Can you work these out from the model? Positions are in its coordinate system, mm. A direction names the side the tool comes from. Round coordinates to 2 decimals unless told otherwise and drop trailing zeros. Order: outer loops, then holes, each group sorted by start corner. A loop starts at its lowest first (then second) coordinate and runs counter-clockwise, first axis right, second up.
Q1. For faces 1 (the face through (16.051, 0.507, -3.636)), 2 (the face through (-3.905, 1.812, -0.867)), 3 (the face through (10, 0, 1)), which set-ups out of +Z, -Z, +X, -X, +Y, -Y let a thin tool reach every point of the face, with its end or its side?
Q2. Will these pins go through, and if not, where does the flat tip stop? P1, Ø1, axis at y = 2, z = 2.5, coming from the -X side; P2, Ø1.5, axis at y = 2.5, z = -3, coming from the -X side; P3, Ø4, axis at x = 9.5, z = 3, coming from the -Y side; P4, Ø1.5, axis at y = 0.5, z = -2, coming from the -X side.
Q3. If we section it at A-A (y = 1.4): Please give me the cut outline in (x, z).
Q4. If we section it at C-C (x = 5.25): Please give me the cut outline in (y, z), plus the area to 3 significant figures.
Q5. If I drill on line 1 (Y direction, x = 7.75, z = 1.5); line 2 (X direction, y = 1.7, z = -0.5); line 3 (Z direction, x = 9.75, y = 0.65), over which ranges is the centre line in solid material (lowest first)?
Q6. We'd pull the mould along X, two halves only. Please class faces 4 (the face through (1.3, 0.5, -4)), 5 (the face through (9.9, 0.5, 0)): pulls with the +X half, pulls with the -X half, needs draft (parallel to the pull), parting line crosses it, or undercut.
Q7. If we section it at B-B (x = 11.75): Please give me the cut outline in (y, z), plus the area to 3 significant figures.
from build123d import *

# Parameters (mm, degrees)
SKETCH1_R             = 4
BOSS_EXTRUDE1_DEPTH   = 4
BOSS_EXTRUDE1_2_DEPTH = 4
FILLET1_R             = 1
FILLET2_R             = 1
SKETCH2_W             = 20
SKETCH2_H             = 8
BOSS_EXTRUDE2_DEPTH   = 1
SKETCH3_R             = 6
CUT_EXTRUDE1_DEPTH    = 1
FILLET3_R             = 3


with BuildPart() as part:
    # Sketch1 → Boss-Extrude1 (new body)
    with BuildSketch(Plane(origin=(0, 0, 0), x_dir=(1, 0, 0), z_dir=(0, 1, 0))):
        with Locations(Location((0, 0, 0), (0, 0, 270))):
            Circle(SKETCH1_R)
    extrude(amount=BOSS_EXTRUDE1_DEPTH)

    # Fillet1
    fillet1_edges = [part.edges().sort_by_distance(p)[0] for p in [
        (0, 4, -4),
    ]]
    fillet(fillet1_edges, radius=FILLET1_R)



with BuildPart() as body_2:
    # Sketch1 → Boss-Extrude1 2 (new body)
    with BuildSketch(Plane(origin=(0, 0, 0), x_dir=(1, 0, 0), z_dir=(0, 1, 0))):
        with Locations(Location((20, 0, 0), (0, 0, 270))):
            Circle(SKETCH1_R)
    extrude(amount=BOSS_EXTRUDE1_2_DEPTH)

    # Fillet2
    fillet2_edges = [body_2.edges().sort_by_distance(p)[0] for p in [
        (20, 4, -4),
    ]]
    fillet(fillet2_edges, radius=FILLET2_R)


with BuildPart() as part_1:
    add(part.part)

    add(body_2.part)  # Boss-Extrude2 merges body 2
    # Sketch2 → Boss-Extrude2 (add)
    with BuildSketch(Plane(origin=(0, 0, 0), x_dir=(-1, 0, 0), z_dir=(0, -1, 0))):
        with Locations((-10, 0)):
            Rectangle(SKETCH2_W, SKETCH2_H)
    extrude(amount=-BOSS_EXTRUDE2_DEPTH)

    # Sketch3 → Cut-Extrude1 (cut)
    with BuildSketch(Plane(origin=(0, 1, 0), x_dir=(1, 0, 0), z_dir=(0, 1, 0))):
        with Locations((10, 6)):
            Circle(SKETCH3_R)
    extrude(amount=-CUT_EXTRUDE1_DEPTH, mode=Mode.SUBTRACT)

    # Fillet3
    fillet3_edges = [part_1.edges().sort_by_distance(p)[0] for p in [
        (4.343145751, 0.5, -4),
        (15.656854249, 0.5, -4),
    ]]
    fillet(fillet3_edges, radius=FILLET3_R)


solid = part_1.part
Solution:
1. face 1: -Z, +Y, -Y
1. face 2: +Y
1. face 3: +Z, -Z, +X, -X, -Y
2. P1: stops at x = -3.46
2. P2: stops at x = -3.31
2. P3: stops at y = 0
2. P4: stops at x = -3.8
3. outline: circle Ø8 at (0, 0); circle Ø8 at (20, 0)
4. outline: (0, -2.33) - (1, -2.33) - (1, 4) - (0, 4) - close
4. area: 6.33 mm2
5. line 1: y = 0 to 1
5. line 2: x = -3.97 to 3.97, 16.03 to 23.97
5. line 3: z = -0.01 to 4
6. face 4: needs draft
6. face 5: undercut
7. outline: (0, -0.26) - (1, -0.26) - (1, 4) - (0, 4) - close
7. area: 4.26 mm2
